Could you check a few things on this model? Use its own coordinates, in mm. Round coordinates to 2 decimals unless told otherwise and drop trailing zeros. Write each loop counter-clockwise with the first axis right and the second up, starting at its lowest first coordinate (ties: lowest second). Pieces come first, ordered by that corner, then holes. Notation, with made-up numbers: (-27.5, -2.5) -> (3.5, -2.5) arc R15 cw to (3.5, 19.5) -> close; hole circle Ø7 at (67, 81). An arc over 180 degrees is marked (long way). One line per question, with ' | ' between items. Start each with the question number.
1. If I drill on line 1 along Y through (x, z) = (0, 3.45); line 2 along Y through (x, z) = (0, 0.5); line 3 along Y through (x, z) = (-10, 1), over which ranges is the centre line in solid material (lowest first)? Write a range as [from, to].
2. Imagine slicing it at C-C, the plane z = 1.75. List the corners of the cut face in (x, y) for me.
3. Imagine slicing it at B-B, the plane y = 75. List the corners of the cut face in (x, z) for me, and give its area (3 significant figures).
4. Imagine slicing it at A-A, the plane x = 0. List the corners of the cut face in (y, z) for me, and give its area (3 significant figures).
from build123d import *

# Parameters (mm, degrees)
SKETCH1_W           = 22
SKETCH1_H           = 170
BOSS_EXTRUDE1_DEPTH = 4
FILLET1_R           = 5
FILLET2_R           = 2
SKETCH2_R           = 5
CUT_EXTRUDE1_DEPTH  = 87.081356867
SKETCH3_R           = 6.75
CUT_EXTRUDE2_DEPTH  = 1


with BuildPart() as part:
    # Sketch1 → Boss-Extrude1 (new, symmetric)
    with BuildSketch(Plane.XY):
        Rectangle(SKETCH1_W, SKETCH1_H)
    extrude(amount=BOSS_EXTRUDE1_DEPTH, both=True)

    # Fillet1
    fillet1_edges = [part.edges().sort_by_distance(p)[0] for p in [
        (11, -85, 0),
        (-11, -85, 0),
        (-11, 85, 0),
        (11, 85, 0),
    ]]
    fillet(fillet1_edges, radius=FILLET1_R)

    # Fillet2
    fillet2_edges = [part.edges().sort_by_distance(p)[0] for p in [
        (11, 0, -4),
        (0, -85, -4),
        (-11, 0, -4),
        (0, 85, -4),
        (9.535533906, 83.535533906, -4),
        (-9.535533906, 83.535533906, -4),
        (-9.535533906, -83.535533906, -4),
        (9.535533906, -83.535533906, -4),
    ]]
    fillet(fillet2_edges, radius=FILLET2_R)

    # Sketch2 → Cut-Extrude1 (cut, through all)
    with BuildSketch(Plane.XY.offset(4)):
        with Locations((0, 75)):
            Circle(SKETCH2_R)
        with Locations((0, -75)):
            Circle(SKETCH2_R)
    extrude(amount=-CUT_EXTRUDE1_DEPTH, mode=Mode.SUBTRACT)

    # Sketch3 → Cut-Extrude2 (cut)
    with BuildSketch(Plane.XY.offset(4)):
        with Locations((0, 75)):
            Circle(SKETCH3_R)
        with Locations((0, -75)):
            Circle(SKETCH3_R)
    extrude(amount=-CUT_EXTRUDE2_DEPTH, mode=Mode.SUBTRACT)


solid = part.part
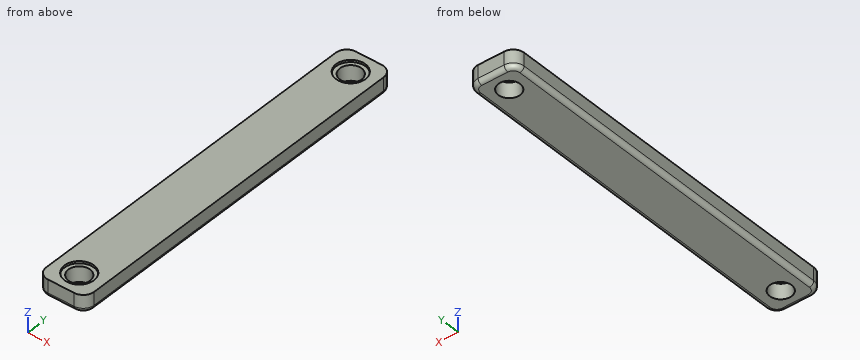
Geometry results:
1) line 1: y = [-85, -81.75], [-68.25, 68.25], [81.75, 85] | line 2: y = [-85, -80], [-70, 70], [80, 85] | line 3: y = [-83, 83]
2) outline: (-11, -80) arc R5 ccw to (-6, -85) -> (6, -85) arc R5 ccw to (11, -80) -> (11, 80) arc R5 ccw to (6, 85) -> (-6, 85) arc R5 ccw to (-11, 80) -> close; hole circle Ø10 at (0, -75); hole circle Ø10 at (0, 75)
3) outline: (-11, -2) arc R2 ccw to (-9, -4) -> (-5, -4) -> (-5, 3) -> (-6.75, 3) -> (-6.75, 4) -> (-11, 4) -> close; (5, -4) -> (9, -4) arc R2 ccw to (11, -2) -> (11, 4) -> (6.75, 4) -> (6.75, 3) -> (5, 3) -> close | area: 90.8 mm2
4) outline: (-85, -2) arc R2 ccw to (-83, -4) -> (-80, -4) -> (-80, 3) -> (-81.75, 3) -> (-81.75, 4) -> (-85, 4) -> close; (-70, -4) -> (70, -4) -> (70, 3) -> (68.25, 3) -> (68.25, 4) -> (-68.25, 4) -> (-68.25, 3) -> (-70, 3) -> close; (80, -4) -> (83, -4) arc R2 ccw to (85, -2) -> (85, 4) -> (81.75, 4) -> (81.75, 3) -> (80, 3) -> close | area: 1,190 mm2
